```python
from build123d import *

# Parameters (mm, degrees)
SKETCH1_W           = 46.3
SKETCH1_H           = 180
BOSS_EXTRUDE1_DEPTH = 6
CUT_EXTRUDE1_REACH  = 187.956
SKETCH2_R           = 8
CUT_EXTRUDE2_REACH  = 187.956
SKETCH4_R           = 1.5
SKETCH4_W           = 20
SKETCH4_H           = 41


with BuildPart() as part:
    # Sketch1 → Boss-Extrude1 (new body)
    with BuildSketch(Plane(origin=(0, 0, 0), x_dir=(1, 0, 0), z_dir=(0, 1, 0))):
        with Locations((23.15, 90)):
            Rectangle(SKETCH1_W, SKETCH1_H)
    extrude(amount=BOSS_EXTRUDE1_DEPTH)

    # Sketch2 → Cut-Extrude1 (cut, up to next)
    with BuildSketch(Plane(origin=(0, 6, 0), x_dir=(1, 0, 0), z_dir=(0, 1, 0)), mode=Mode.PRIVATE) as cut_extrude1_sk1:
        with Locations(Location((23.15, 18.5, 0), (0, 0, 270))):
            Circle(SKETCH2_R)
    cut_extrude1_tool1 = extrude(cut_extrude1_sk1.sketch, amount=-CUT_EXTRUDE1_REACH, mode=Mode.PRIVATE) & part.part
    add(cut_extrude1_tool1.solids().sort_by_distance((23.15, 6, -18.5))[0], mode=Mode.SUBTRACT)

    # Sketch4 → Cut-Extrude2 (cut, up to next)
    with BuildSketch(Plane.XZ, mode=Mode.PRIVATE) as cut_extrude2_sk1:
        with Locations(Location((28.15, -173.5, 0), (0, 0, 270))):
            Circle(SKETCH4_R)
    cut_extrude2_tool1 = extrude(cut_extrude2_sk1.sketch, amount=-CUT_EXTRUDE2_REACH, mode=Mode.PRIVATE) & part.part
    # Sketch4 → Cut-Extrude2 (cut, up to next)
    with BuildSketch(Plane.XZ, mode=Mode.PRIVATE) as cut_extrude2_sk2:
        with Locations(Location((18.15, -173.5, 0), (0, 0, 270))):
            Circle(SKETCH4_R)
    cut_extrude2_tool2 = extrude(cut_extrude2_sk2.sketch, amount=-CUT_EXTRUDE2_REACH, mode=Mode.PRIVATE) & part.part
    # Sketch4 → Cut-Extrude2 (cut, up to next)
    with BuildSketch(Plane.XZ, mode=Mode.PRIVATE) as cut_extrude2_sk3:
        with Locations(Location((18.15, -125.5, 0), (0, 0, 270))):
            Circle(SKETCH4_R)
    cut_extrude2_tool3 = extrude(cut_extrude2_sk3.sketch, amount=-CUT_EXTRUDE2_REACH, mode=Mode.PRIVATE) & part.part
    # Sketch4 → Cut-Extrude2 (cut, up to next)
    with BuildSketch(Plane.XZ, mode=Mode.PRIVATE) as cut_extrude2_sk4:
        with Locations(Location((28.15, -125.5, 0), (0, 0, 270))):
            Circle(SKETCH4_R)
    cut_extrude2_tool4 = extrude(cut_extrude2_sk4.sketch, amount=-CUT_EXTRUDE2_REACH, mode=Mode.PRIVATE) & part.part
    # Sketch4 → Cut-Extrude2 (cut, up to next)
    with BuildSketch(Plane.XZ, mode=Mode.PRIVATE) as cut_extrude2_sk5:
        with Locations((23.15, -149.5)):
            Rectangle(SKETCH4_W, SKETCH4_H)
    cut_extrude2_tool5 = extrude(cut_extrude2_sk5.sketch, amount=-CUT_EXTRUDE2_REACH, mode=Mode.PRIVATE) & part.part
    add(cut_extrude2_tool1.solids().sort_by_distance((28.15, 0, -173.5))[0], mode=Mode.SUBTRACT)
    add(cut_extrude2_tool2.solids().sort_by_distance((18.15, 0, -173.5))[0], mode=Mode.SUBTRACT)
    add(cut_extrude2_tool3.solids().sort_by_distance((18.15, 0, -125.5))[0], mode=Mode.SUBTRACT)
    add(cut_extrude2_tool4.solids().sort_by_distance((28.15, 0, -125.5))[0], mode=Mode.SUBTRACT)
    add(cut_extrude2_tool5.solids().sort_by_distance((23.15, 0, -149.5))[0], mode=Mode.SUBTRACT)


solid = part.part
```
Verification items for the finished model (mm, model axes). A direction names the side the tool comes from. Give positions to 0.01 mm unless a question says otherwise; leave off trailing zeros. Order: outer loops, then holes, each group sorted by start corner. A loop starts at its lowest first (then second) coordinate and runs counter-clockwise, first axis right, second up. Notation, with made-up numbers: M -24,-2 L 3,-2 A15 cw 3,13 Z; hole C -12,74 d11. An arc over 180 degrees is marked long. Answer in a Markdown table with one row per item. Add a question column.
Item 1: Gauge pin test, flat end, axial feed: pin 1 (14.5 mm diameter, centred on x = 23.15, z = -18.5, fed in from +Y). Record the tip position at first contact, or that the pin passes through.
Item 2: Section check A-A, the plane x = 23.15. Enter the section's corners in (y, z).
Item 3: Section check C-C, the plane y = 3.9. Enter the section's corners in (x, z).
Item 4: Section check B-B, the plane z = -125.5. Enter the section's corners in (x, y).
Item 5: Mould release check, pull along X, two halves, no side actions. Record for faces 3 (the flat face through (46.3, 3, -89)), 4 (the flat face through (0, 3, -89)), 5 (the flat face through (13.15, 3, -150)), 6 (the flat face through (23, 3, -180)): released by +X, released by -X, zero draft, split by the parting line, or undercut.
Item 6: Scan lines: probe 1 along X at (y, z) = (3.8, -173.5); probe 2 along X at (y, z) = (1.45, -18.5); probe 3 along X at (y, z) = (5.65, -138). Record each from-to range of solid material in increasing order. Write a range as from..to.
Item 7: Tool access check on faces 1 (the flat face through (23, 3, -129)), 2 (the flat face through (23, 3, 0)). Record the directions out of +Z, -Z, +X, -X, +Y, -Y that give a thin tool (end or side, any length) a straight path to the whole face; none if there is none.
Filled sheet:
| question | item | result |
|---|---|---|
| 1 | pin 1 | passes through |
| 2 | outline | M 0,-180 L 6,-180 L 6,-170 L 0,-170 Z; M 0,-129 L 6,-129 L 6,-26.5 L 0,-26.5 Z; M 0,-10.5 L 6,-10.5 L 6,0 L 0,0 Z |
| 3 | outline | M 0,-180 L 46.3,-180 L 46.3,0 L 0,0 Z; hole M 13.15,-170 L 33.15,-170 L 33.15,-129 L 13.15,-129 Z; hole C 23.15,-18.5 d16; hole C 18.15,-173.5 d3; hole C 18.15,-125.5 d3; hole C 28.15,-173.5 d3; hole C 28.15,-125.5 d3 |
| 4 | outline | M 0,0 L 16.65,0 L 16.65,6 L 0,6 Z; M 19.65,0 L 26.65,0 L 26.65,6 L 19.65,6 Z; M 29.65,0 L 46.3,0 L 46.3,6 L 29.65,6 Z |
| 5 | face 3 | released by +X |
| 5 | face 4 | released by -X |
| 5 | face 5 | undercut |
| 5 | face 6 | zero draft |
| 6 | probe 1 | x = 0..16.65, 19.65..26.65, 29.65..46.3 |
| 6 | probe 2 | x = 0..15.15, 31.15..46.3 |
| 6 | probe 3 | x = 0..13.15, 33.15..46.3 |
| 7 | face 1 | +Y, -Y |
| 7 | face 2 | +Z, +X, -X, +Y, -Y |
